Check sheet for the modelled part. Datum: model origin and axes. Units: mm. A direction names the side the tool comes from. Give positions to 0.01 mm unless a question says otherwise; leave off trailing zeros. Order: outer loops, then holes, each group sorted by start corner. A loop starts at its lowest first (then second) coordinate and runs counter-clockwise, first axis right, second up. Notation, with made-up numbers: (-6.5, 28) - (51.5, 28) arc R15 cw to (51.5, 37) - close; hole circle Ø6 at (21, 29). An arc over 180 degrees is marked (long way). Answer in a Markdown table with one row per item.
from build123d import *

# Parameters (mm, degrees)
SKETCH_1_W          = 250
SKETCH_1_H          = 260
EXTRUDE_1_DEPTH     = 1.5
SKETCH_2_W          = 10
SKETCH_2_H          = 10
CUT_EXTRUDE_1_DEPTH = 5
SKETCH_3_R          = 1.25
CUT_EXTRUDE_2_DEPTH = 5
SKETCH_4_R          = 1.25
CUT_EXTRUDE_3_DEPTH = 5
CUT_EXTRUDE_4_DEPTH = 5
CUT_EXTRUDE_5_DEPTH = 5
EXTRUDE_2_DEPTH     = 3
SKETCH_9_R          = 1.5
CUT_EXTRUDE_7_DEPTH = 10
FILLET_1_R          = 2
SKETCH_10_R         = 1.5
CUT_EXTRUDE_8_DEPTH = 10


with BuildPart() as part:
    # 草图1 → 凸台-拉伸1 (new, symmetric)
    with BuildSketch(Plane.XY):
        Rectangle(SKETCH_1_W, SKETCH_1_H)
    extrude(amount=EXTRUDE_1_DEPTH, both=True)

    # 草图2 → 切除-拉伸1 (cut, symmetric)
    with BuildSketch(Plane(origin=(0, 0, -1.5), x_dir=(-1, 0, 0), z_dir=(0, 0, -1))):
        with Locations((50, -110)):
            Rectangle(SKETCH_2_W, SKETCH_2_H)
        with Locations((-50, 110)):
            Rectangle(SKETCH_2_W, SKETCH_2_H)
        with Locations((50, 110)):
            Rectangle(SKETCH_2_W, SKETCH_2_H)
        with Locations((110, 55)):
            Rectangle(SKETCH_2_W, SKETCH_2_H)
        with Locations((110, -55)):
            Rectangle(SKETCH_2_W, SKETCH_2_H)
        with Locations((-50, -110)):
            Rectangle(SKETCH_2_W, SKETCH_2_H)
        with Locations((-110, 55)):
            Rectangle(SKETCH_2_W, SKETCH_2_H)
        with Locations((-110, -55)):
            Rectangle(SKETCH_2_W, SKETCH_2_H)
    extrude(amount=CUT_EXTRUDE_1_DEPTH, both=True, mode=Mode.SUBTRACT)

    # 草图3 → 切除-拉伸2 (cut, symmetric)
    with BuildSketch(Plane(origin=(0, 0, -1.5), x_dir=(-1, 0, 0), z_dir=(0, 0, -1))):
        with Locations((-55, 113.75)):
            Circle(SKETCH_3_R)
        with Locations((-55, 106.25)):
            Circle(SKETCH_3_R)
        with Locations((-45, 106.25)):
            Circle(SKETCH_3_R)
        with Locations((-45, 113.75)):
            Circle(SKETCH_3_R)
        with Locations((45, 113.75)):
            Circle(SKETCH_3_R)
        with Locations((45, 106.25)):
            Circle(SKETCH_3_R)
        with Locations((55, 106.25)):
            Circle(SKETCH_3_R)
        with Locations((55, 113.75)):
            Circle(SKETCH_3_R)
    cut_extrude_2 = extrude(amount=CUT_EXTRUDE_2_DEPTH, both=True, mode=Mode.SUBTRACT)

    # 草图4 → 切除-拉伸3 (cut, symmetric)
    with BuildSketch(Plane(origin=(0, 0, -1.5), x_dir=(-1, 0, 0), z_dir=(0, 0, -1))):
        with Locations((106.25, 60)):
            Circle(SKETCH_4_R)
        with Locations((113.75, 60)):
            Circle(SKETCH_4_R)
        with Locations((106.25, 50)):
            Circle(SKETCH_4_R)
        with Locations((113.75, 50)):
            Circle(SKETCH_4_R)
        with Locations((113.75, -50)):
            Circle(SKETCH_4_R)
        with Locations((106.25, -50)):
            Circle(SKETCH_4_R)
        with Locations((113.75, -60)):
            Circle(SKETCH_4_R)
        with Locations((106.25, -60)):
            Circle(SKETCH_4_R)
    cut_extrude_3 = extrude(amount=CUT_EXTRUDE_3_DEPTH, both=True, mode=Mode.SUBTRACT)

    # 镜向1: 切除-拉伸3 across plane
    add(cut_extrude_3.mirror(Plane(origin=(0, 0, 0), x_dir=(0, 0, 1), z_dir=(1, 0, 0))), mode=Mode.SUBTRACT)

    # 镜向2: 切除-拉伸2 across plane
    add(cut_extrude_2.mirror(Plane.ZX), mode=Mode.SUBTRACT)

    # 草图5 → 切除-拉伸4 (cut, symmetric)
    with BuildSketch(Plane(origin=(0, 0, -1.5), x_dir=(-1, 0, 0), z_dir=(0, 0, -1))):
        Polygon((-60, 130), (-125, 65), (-125, 130), align=None)
        Polygon((-125, -130), (-60, -130), (-125, -65), align=None)
    cut_extrude_4 = extrude(amount=CUT_EXTRUDE_4_DEPTH, both=True, mode=Mode.SUBTRACT)

    # 镜向3: 切除-拉伸4 across plane
    add(cut_extrude_4.mirror(Plane(origin=(0, 0, 0), x_dir=(0, 0, 1), z_dir=(1, 0, 0))), mode=Mode.SUBTRACT)

    # 草图6 → 切除-拉伸5 (cut, symmetric)
    with BuildSketch(Plane(origin=(0, 0, -1.5), x_dir=(-1, 0, 0), z_dir=(0, 0, -1))):
        Polygon((95, -52.573593129), (95, 52.573593129), (47.573593129, 100), (-47.573593129, 100), (-95, 52.573593129), (-95, -52.573593129), (-47.573593129, -100), (47.573593129, -100), align=None)
    extrude(amount=CUT_EXTRUDE_5_DEPTH, both=True, mode=Mode.SUBTRACT)

    # 草图7 → 凸台-拉伸2 (add)
    with BuildSketch(Plane(origin=(0, 0, -1.5), x_dir=(-1, 0, 0), z_dir=(0, 0, -1))):
        Polygon((-51.185672274, 98.281604164), (-8.964661116, 9.532766034), (-93.063178997, 56.073410896), (-96.936821003, 49.073775362), (-8.260959569, 0), (-96.936821003, -49.073775362), (-93.063178997, -56.073410896), (-8.964661116, -9.532766034), (-51.185672274, -98.281604164), (-43.961513984, -101.718395836), (0, -9.311009527), (43.961513984, -101.718395836), (51.185672274, -98.281604164), (8.964661116, -9.532766034), (93.063178997, -56.073410896), (96.936821003, -49.073775362), (8.260959569, 0), (96.936821003, 49.073775362), (93.063178997, 56.073410896), (8.964661116, 9.532766034), (51.185672274, 98.281604164), (43.961513984, 101.718395836), (0, 9.311009527), (-43.961513984, 101.718395836), align=None)
    extrude(amount=-EXTRUDE_2_DEPTH)

    # 草图9 → 切除-拉伸7 (cut)
    with BuildSketch(Plane(origin=(0, 0, -1.5), x_dir=(-1, 0, 0), z_dir=(0, 0, -1))):
        with Locations((70, 38.738437042)):
            Circle(SKETCH_9_R)
        with Locations((70, 98.738437042)):
            Circle(SKETCH_9_R)
        with Locations((70, -98.738437042)):
            Circle(SKETCH_9_R)
        with Locations((70, -38.738437042)):
            Circle(SKETCH_9_R)
    cut_extrude_7 = extrude(amount=-CUT_EXTRUDE_7_DEPTH, mode=Mode.SUBTRACT)

    # 镜向4: 切除-拉伸7 across plane
    add(cut_extrude_7.mirror(Plane(origin=(0, 0, 0), x_dir=(0, 0, 1), z_dir=(1, 0, 0))), mode=Mode.SUBTRACT)

    # 圆角1
    fillet_1_edges = [part.edges().sort_by_distance(p)[0] for p in [
        (-95, -48.001926526, 0),
        (-95, 48.001926526, 0),
        (-92.057005132, 55.516587997, 0),
        (-50.575201814, 96.998391315, 0),
        (-43.14401134, 100, 0),
        (43.14401134, 100, 0),
        (50.575201814, 96.998391315, 0),
        (92.057005132, 55.516587997, 0),
        (95, 48.001926526, 0),
        (95, -48.001926526, 0),
        (92.057005132, -55.516587997, 0),
        (50.575201814, -96.998391315, 0),
        (43.14401134, -100, 0),
        (-43.14401134, -100, 0),
        (-50.575201814, -96.998391315, 0),
        (-92.057005132, -55.516587997, 0),
        (-8.964661116, -9.532766034, 0),
        (0, -9.311009527, 0),
        (8.964661116, -9.532766034, 0),
        (8.260959569, 0, 0),
        (8.964661116, 9.532766034, 0),
        (0, 9.311009527, 0),
        (-8.964661116, 9.532766034, 0),
        (-8.260959569, 0, 0),
    ]]
    fillet(fillet_1_edges, radius=FILLET_1_R)

    # 草图10 → 切除-拉伸8 (cut)
    with BuildSketch(Plane(origin=(0, 0, -1.5), x_dir=(-1, 0, 0), z_dir=(0, 0, -1))):
        with Locations((36.869534675, 77.5)):
            Circle(SKETCH_10_R)
        with Locations((-36.869534675, 77.5)):
            Circle(SKETCH_10_R)
        with Locations((-36.869534675, -77.5)):
            Circle(SKETCH_10_R)
        with Locations((36.869534675, -77.5)):
            Circle(SKETCH_10_R)
    extrude(amount=-CUT_EXTRUDE_8_DEPTH, mode=Mode.SUBTRACT)


solid = part.part
(1) Mould release check, pull along X, two halves, no side actions. Record for faces 1 (the flat face through (-10, 1, 1.5)), 2 (the flat face through (51.55, 33.1, -0.02)), 3 (the flat face through (-92, 98, 0)): pulls with the +X half, pulls with the -X half, needs draft (parallel to the pull), parting line crosses it, or undercut.
Geometry says:
| item | result |
|---|---|
| face 1 | needs draft |
| face 2 | undercut |
| face 3 | pulls with the -X half |
(2) Gauge pin test, flat ends, axial feed: P1, Ø2.5, axis at x = 70, y = -38.74, coming from the -Z side; P2, Ø0.9, axis at x = -111, z = -0.5, coming from the +Y side. Record the tip position at first contact, or that the pin passes through.
Geometry says:
| item | result |
|---|---|
| P1 | through |
| P2 | y = 79.45 |
(3) Access from +Z, -Z, +X, -X, +Y, -Y to the whole of each face (thin tool, end or side, straight path). Record for faces 4 (the flat face through (92, -98, 0)), 5 (the flat face through (51.16, -23.74, -0.02)).
Geometry says:
| item | result |
|---|---|
| face 4 | +Z, -Z, +X, -Y |
| face 5 | +Z, -Z |
(4) Cross-section at C-C, the plane z = -0.8. Give the number of separate pieces and of enclosed holes in the cut face, then the cut area to 3 significant figures.
Geometry says:
| item | result |
|---|---|
| separate pieces | 1 |
| enclosed holes | 28 |
| area | 28,800 mm² |
(5) Cross-section at B-B, the plane x = -20. Record the cut outline in (y, z), then the cut area to 3 significant figures.
Geometry says:
| item | result |
|---|---|
| outline | (-130, -1.5) - (-100, -1.5) - (-100, 1.5) - (-130, 1.5) - close; (-51.35, -1.5) - (-32.73, -1.5) - (-32.73, 1.5) - (-51.35, 1.5) - close; (-15.64, -1.5) - (-6.5, -1.5) - (-6.5, 1.5) - (-15.64, 1.5) - close; (6.5, -1.5) - (15.64, -1.5) - (15.64, 1.5) - (6.5, 1.5) - close; (32.73, -1.5) - (51.35, -1.5) - (51.35, 1.5) - (32.73, 1.5) - close; (100, -1.5) - (130, -1.5) - (130, 1.5) - (100, 1.5) - close |
| area | 347 mm² |
(6) Thickness scan on L1, parallel to X at y = -67, z = -0.3; L2, parallel to X at y = 93, z = 0.95; L3, parallel to X at y = 2.5, z = -0.45. Record the ranges inside material, lowest first.
Geometry says:
| item | result |
|---|---|
| L1 | -123 to -80.57, -36.3 to -27.44, 27.44 to 36.3, 80.57 to 123 |
| L2 | -97 to -54.57, -48.67 to -39.81, 39.81 to 48.67, 54.57 to 97 |
| L3 | -125 to -95, -12.78 to 12.78, 95 to 125 |
(7) Cross-section at A-A, the plane x = -80.5. Record the cut outline in (y, z).
Geometry says:
| item | result |
|---|---|
| outline | (-109.5, -1.5) - (-67.07, -1.5) - (-67.07, 1.5) - (-109.5, 1.5) - close; (-49.12, -1.5) - (-39.98, -1.5) - (-39.98, 1.5) - (-49.12, 1.5) - close; (39.98, -1.5) - (49.12, -1.5) - (49.12, 1.5) - (39.98, 1.5) - close; (67.07, -1.5) - (109.5, -1.5) - (109.5, 1.5) - (67.07, 1.5) - close |
